Build history of the part. All positions in model axes, mm. Face numbers are marked on the shaded views. A direction names the side the tool comes from. Give positions to 0.01 mm unless a question says otherwise; leave off trailing zeros. Order: outer loops, then holes, each group sorted by start corner. A loop starts at its lowest first (then second) coordinate and runs counter-clockwise, first axis right, second up. Notation, with made-up numbers: (-36.75, 77) - (12.25, 77) arc R27 cw to (12.25, 99) - close; hole circle Ø10 at (4, 30). An arc over 180 degrees is marked (long way). Use a Markdown table: item, result. Add a question column.
(1) Slice it at B-B (x = 5.5). Write the cut outline in (y, z), then the cut area to 3 significant figures.
(2) Slice it at C-C (z = -2.5). Write the cut outline in (x, y), then the cut area to 3 significant figures.
(3) Mould opens along Z. For the marked faces 3, 4, 5 and 6 say: +Z half, -Z half, draft (parallel to the pull), parting line (faces both ways), or undercut.
(4) Flat gauge pin, fed straight in: pin 1 (9 mm diameter, centred on x = 6, z = -2.5, fed in from -Y). Where does the tip first touch, or does it go through?
(5) Slice it at A-A (y = -15.25). Write the cut outline in (x, z).
(6) Which spindle directions (+Z, -Z, +X, -X, +Y, -Y) get a long thin tool onto all of the face, cutting with end or side? Do the marked faces 1 and 2. Say none if no direction does.
(7) Wall check: line 1 (Z direction, x = -12.75, y = -4.25); line 2 (Y direction, x = -10.25, z = -9). Give the ranges that are in metal, low to high.
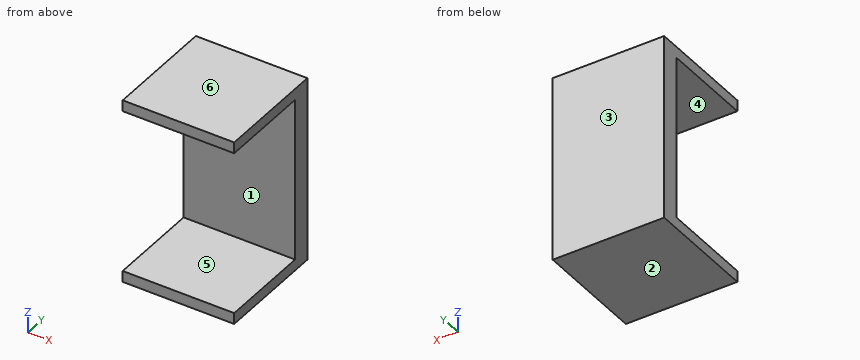
from build123d import *

# Parameters (mm, degrees)
F1_DEPTH = 15


with BuildPart() as f1:
    # F0 (on Right) → F1 (new body, symmetric)
    with BuildSketch(Plane.YZ):
        Polygon((0, -1.8719722131), (-30, -1.8719722131), (-30, -4.8719722131), (-5, -4.8719722131), (-5, -48.8719722131), (-30, -48.8719722131), (-30, -51.8719722131), (0, -51.8719722131), align=None)
    extrude(amount=F1_DEPTH, both=True)


with BuildPart() as f1_1:
    # F2: moved
    add(f1.part.moved(Location((0, 3.7136785686, 28.4729581326))))


solid = f1_1.part
Solution:
| question | item | result |
|---|---|---|
| 1 | outline | (-26.29, -23.4) - (3.71, -23.4) - (3.71, 26.6) - (-26.29, 26.6) - (-26.29, 23.6) - (-1.29, 23.6) - (-1.29, -20.4) - (-26.29, -20.4) - close |
| 1 | area | 400 mm2 |
| 2 | outline | (-15, -1.29) - (15, -1.29) - (15, 3.71) - (-15, 3.71) - close |
| 2 | area | 150 mm2 |
| 3 | face 3 | draft |
| 3 | face 4 | undercut |
| 3 | face 5 | undercut |
| 3 | face 6 | +Z half |
| 4 | pin 1 | y = -1.29 |
| 5 | outline | (-15, -23.4) - (15, -23.4) - (15, -20.4) - (-15, -20.4) - close; (-15, 23.6) - (15, 23.6) - (15, 26.6) - (-15, 26.6) - close |
| 6 | face 1 | +X, -X, -Y |
| 6 | face 2 | -Z, +X, -X, +Y, -Y |
| 7 | line 1 | -23.4 to -20.4, 23.6 to 26.6 |
| 7 | line 2 | -1.29 to 3.71 |
